Work out the finished part from the listing and answer in its coordinate system (mm). A direction names the side the tool comes from. Round coordinates to 2 decimals unless told otherwise and drop trailing zeros. Answer as a JSON object with one key per item and string values.
```python
from build123d import *

# Parameters (mm, degrees)
F0_W     = 63.5
F0_H     = 19.05
F1_DEPTH = 8.89
F2_R     = 3.81


with BuildPart() as f1:
    # F0 (on Top) → F1 (new body)
    with BuildSketch(Plane.XY):
        with Locations((31.75, 9.525)):
            Rectangle(F0_W, F0_H)
        Polygon((3.857002, 9.525), (5.103501, 11.684), (7.596499, 11.684), (8.842998, 9.525), (7.596499, 7.366), (5.103501, 7.366), align=None, mode=Mode.SUBTRACT)
        Polygon((54.657002, 9.525), (55.903501, 11.684), (58.396499, 11.684), (59.642998, 9.525), (58.396499, 7.366), (55.903501, 7.366), align=None, mode=Mode.SUBTRACT)
    extrude(amount=F1_DEPTH)

    # F2
    f2_edges = [f1.edges().sort_by_distance(p)[0] for p in [
        (0, 0, 4.445),
        (0, 19.05, 4.445),
        (63.5, 0, 4.445),
        (63.5, 19.05, 4.445),
    ]]
    fillet(f2_edges, radius=F2_R)


solid = f1.part
```
Item 1: Consider line 1 along X through (y, z) = (11, 4); line 2 along X through (y, z) = (8.25, 4.5); line 3 along Y through (x, z) = (60, 5.25). Determine where each line is inside the solid, lowest interval first.
Results found:
{"line 1": "0 to 4.71, 7.99 to 55.51, 58.79 to 63.5", "line 2": "0 to 4.59, 8.11 to 55.39, 58.91 to 63.5", "line 3": "0.01 to 19.04"}
Item 2: This flat-tipped pin is pushed along its axis until it touches: P1, Ø2, axis at y = 2.5, z = 5, coming from the -X side. Where does it stop, or does it pass through?
Results found:
{"P1": "x = 0.01"}
Item 3: A cutting plane is placed at A-A (z = 3.5). Give the number of separate pieces and of enclosed holes in the cut face, and give its area (3 significant figures).
Results found:
{"separate pieces": "1", "enclosed holes": "2", "area": "1,160 mm²"}
Item 4: For faces 1 (the flat face through (31, 0, 4)), 2 (the flat face through (4.49, 8.43, 4.38)), determine the directions among +Z, -Z, +X, -X, +Y, -Y from which every point of the face is accessible in a straight line to the end or side of a thin tool.
Results found:
{"face 1": "+Z, -Z, +X, -X, -Y", "face 2": "+Z, -Z"}
Item 5: Determine the mould class of faces 3 (the flat face through (8.21, 10.62, 4.38)), 4 (the cylindrical face through (62.354, 17.964, 4.507)), 5 (the flat face through (31, 10, 0)) for opening direction X: pulls with the +X half, pulls with the -X half, needs draft (parallel to the pull), parting line crosses it, or undercut.
Results found:
{"face 3": "undercut", "face 4": "pulls with the +X half", "face 5": "needs draft"}
